Build history of the part. All positions in model axes, mm. A direction names the side the tool comes from. Round coordinates to 2 decimals unless told otherwise and drop trailing zeros. Write each loop counter-clockwise with the first axis right and the second up, starting at its lowest first coordinate (ties: lowest second). Pieces come first, ordered by that corner, then holes. Notation, with made-up numbers: M 30.25,32 L 59.25,32 A19 ccw 59.25,49 Z; hole C 5,88 d7. An arc over 180 degrees is marked long. Use a Markdown table: item, result.
Autodesk Inventor part; units mm, degrees
ref_plane "YZ Plane" through (0, 0, 0) normal (1, 0, 0) x (0, 1, 0)
ref_plane "XZ Plane" through (0, 0, 0) normal (0, 1, 0) x (-1, 0, 0)
ref_plane "XY Plane" through (0, 0, 0) normal (0, 0, 1) x (1, 0, 0)
sketch "スケッチ1" plane through (0, 0, 0) normal (0, 0, 1) x (1, 0, 0)
  line L0 (-24.2059, 21.7891) -> (-24.2059, -29.3158)
  line L1 (-24.2059, -29.3158) -> (21.4201, -29.3158)
  line L2 (21.4196, -22.9707) -> (21.4201, -22.9707)
  line L3 (-11.4832, -22.9707) -> (8.6224, -22.9707)
  arc A0 (-11.4832, -22.9707) -> (-19.2289, -15.2115) centre (-24.2804, -28) ccw
  line L4 (-19.2289, -15.2115) -> (-19.2289, -7.8183)
  arc A1 (-17.2289, -5.8183) -> (-19.2289, -7.8183) centre (-17.2289, -7.8183) ccw
  line L5 (-17.2289, -5.8183) -> (-11.461, -5.8183)
  arc A2 (-11.461, -5.8183) -> (-9.461, -3.8183) centre (-11.461, -3.8183) ccw
  line L6 (-9.461, -3.8183) -> (-9.461, 11.1956)
  arc A3 (-8.461, 12.1956) -> (-9.461, 11.1956) centre (-8.461, 11.1956) ccw
  line L7 (-8.461, 12.1956) -> (5.6023, 12.1956)
  arc A4 (6.6023, 11.1956) -> (5.6023, 12.1956) centre (5.6023, 11.1956) ccw
  line L8 (6.6023, 11.1956) -> (6.6023, -3.8183)
  arc A5 (6.6023, -3.8183) -> (8.6023, -5.8183) centre (8.6023, -3.8183) ccw
  line L9 (8.6023, -5.8183) -> (14.3681, -5.8183)
  arc A6 (16.3681, -7.8183) -> (14.3681, -5.8183) centre (14.3681, -7.8183) ccw
  line L10 (16.3681, -7.8183) -> (16.3681, -15.2115)
  arc A7 (16.3681, -15.2115) -> (8.6224, -22.9707) centre (21.4196, -28) ccw
  circle A8 centre (13.0661, -20.6138) radius 0.954
  circle A9 centre (-15.8899, -20.6138) radius 0.954
  arc A10 (-13.9359, 14.1081) -> (-14.9359, 13.1081) centre (-13.9359, 13.1081) ccw
  line L11 (-14.9359, 13.1081) -> (-14.9359, -0.6888)
  line L12 (-14.9359, -0.6888) -> (-19.2289, -0.6888)
  arc A11 (-5.7797, 14.1081) -> (-4.7797, 15.1081) centre (-5.7797, 15.1081) ccw
  line L13 (-5.7797, 14.1081) -> (-13.9359, 14.1081)
  line L14 (-24.2059, 26.7891) -> (-24.2059, 21.7891)
  line L15 (21.4201, -29.3158) -> (-24.2059, -29.3158)
  line L16 (-24.2059, -29.3158) -> (-24.2059, 26.7891)
  line L17 (21.4196, 26.7891) -> (21.4201, 26.7891)
  line L18 (-24.2059, 36.7891) -> (-24.2059, 26.7891)
  line L19 (-19.2289, 36.7891) -> (-24.2059, 36.7891)
  line L20 (-19.2289, 36.7891) -> (-19.2289, -0.6888)
  line L21 (-4.7797, 15.1081) -> (-4.7797, 36.7891)
  line L22 (21.4201, -29.3158) -> (21.4201, 36.7891)
  line L23 (21.4201, 36.7891) -> (-4.7797, 36.7891)
  line L24 (11.6885, 21.2661) -> (16.9518, 21.2661)
  line L25 (16.9518, 21.2661) -> (16.9518, -1.2633)
  line L26 (16.9518, -1.2633) -> (11.6885, -1.2633)
  line L27 (11.6885, -1.2633) -> (11.6885, 21.2661)
  point P0 (0, 0)
  point P1 (0, 0)
extrude "押し出し1" add sketch "スケッチ1" along normal blind 5
sketch "スケッチ2" plane through (0, 0, 0) normal (0, 0, -1) x (-1, 0, 0)
  line L0 (24.2059, 36.7891) -> (24.2059, -29.3158)
  line L1 (-21.4201, 36.7891) -> (24.2059, 36.7891)
  line L2 (24.2059, 36.7891) -> (24.2059, 31.7891)
  line L3 (24.2059, 31.7891) -> (-21.4201, 31.7891)
  line L4 (-21.4201, 31.7891) -> (-21.4201, 36.7891)
  point P0 (0, 0)
  dimension "d4" = 5
extrude "押し出し2" add sketch "スケッチ2" along normal blind 20
sketch "スケッチ3" plane through (-4.7797, 36.7891, 5) normal (0, 1, 0) x (1, 0, 0)
  line L0 (-10.1561, 5) -> (-14.4492, 5)
  line L1 (-14.4492, 5) -> (0, 5)
  line L2 (0, 5) -> (0, 12)
  line L3 (0, 12) -> (-14.4492, 12)
  line L4 (-14.4492, 12) -> (-14.4492, 5)
  point P0 (4.7797, 5)
  dimension "d7" = 7
extrude "押し出し3" cut sketch "スケッチ3" against normal blind 20
sketch "スケッチ4" plane through (-4.7797, 36.7891, 5) normal (0, 1, 0) x (1, 0, 0)
  circle A0 centre (-14.9262, 21) radius 1.75
  line L0 (-19.4262, 25) -> (26.1998, 25)
  line L1 (-19.4262, 25) -> (-19.4262, 0)
  circle A1 centre (21.6998, 21) radius 1.75
  line L2 (26.1998, 25) -> (26.1998, 0)
  circle A2 centre (21.6998, 15) radius 1.75
  circle A3 centre (-14.9262, 15) radius 1.75
  point P0 (4.7797, 5)
  dimension "d10" = 3.5
  dimension "d11" = 4
  dimension "d12" = 4.5
  dimension "d13" = 3.5
  dimension "d14" = 4
  dimension "d15" = 4.5
  dimension "d16" = 3.5
  dimension "d17" = 6
  dimension "d18" = 3.5
fillet "フィレット1" radius 2 2 edges at (-24.2059, -29.3158, 2.5) (21.4201, -29.3158, 2.5)
extrude "押し出し4" cut sketch "スケッチ4" against normal blind 20
chamfer "面取り1" distance 2 angle 45 2 edges at (8.3202, 31.7891, 0) (-21.7174, 31.7891, 0)
sketch "スケッチ5" plane through (-4.7797, 36.7891, 5) normal (0, 1, 0) x (1, 0, 0)
  circle A0 centre (21.6998, 15) radius 1.75
  circle A1 centre (-14.9262, 21) radius 1.75
  circle A2 centre (21.6998, 21) radius 1.75
  circle A3 centre (-14.9262, 15) radius 1.75
  line L0 (-14.4492, 12) -> (-14.4492, 0)
  line L1 (-14.4492, 12) -> (0, 12)
  line L2 (0, 12) -> (0, 0)
  line L3 (26.1998, 0) -> (0, 0)
  line L4 (26.1998, 25) -> (26.1998, 0)
  line L5 (-19.4262, 25) -> (26.1998, 25)
  line L6 (-19.4262, 25) -> (-19.4262, 0)
  line L7 (-14.4492, 0) -> (-19.4262, 0)
  point P0 (4.7797, 5)
properties part number "OpenMV-Mount-v2"
Q1. Cut at A-A on z = -10. Give the cut face in (x, y), and give its area (3 significant figures).
Response values:
| item | result |
|---|---|
| outline | M -24.21,31.79 L -21.46,31.79 L -21.46,36.79 L -24.21,36.79 Z; M -17.96,31.79 L 15.17,31.79 L 15.17,36.79 L -17.96,36.79 Z; M 18.67,31.79 L 21.42,31.79 L 21.42,36.79 L 18.67,36.79 Z |
| area | 193 mm2 |
Q2. Which spindle directions (+Z, -Z, +X, -X, +Y, -Y) get a long thin tool onto all of the face, cutting with end or side? Do faces 5 (the cylindrical face through (18.59, 34.32, -10.53)), 6 (the flat face through (-19.229, 18, 2)), 7 (the flat face through (16.368, -11, 2)), 8 (the flat face through (8, 1, 0)). Say none if no direction does.
Response values:
| item | result |
|---|---|
| face 5 | +Y, -Y |
| face 6 | +Z, +Y |
| face 7 | +Z, -Z |
| face 8 | -Z, +X, -X, -Y |
Q3. Two-plate mould, pull along Y, no slides. Class faces 1 (the flat face through (16.952, 10, 2)), 2 (the flat face through (-24.206, 14, 1)), 3 (the flat face through (14, 21.266, 2)), 4 (the flat face through (-21.68, 30.8, -1.01)): +Y half, -Y half, draft (parallel to the pull), parting line (faces both ways), or undercut.
Response values:
| item | result |
|---|---|
| face 1 | undercut |
| face 2 | draft |
| face 3 | undercut |
| face 4 | -Y half |
Q4. Cut at B-B on y = -13. Give the cut face in (x, z).
Response values:
| item | result |
|---|---|
| outline | M -24.21,0 L -19.23,0 L -19.23,5 L -24.21,5 Z; M 16.37,0 L 21.42,0 L 21.42,5 L 16.37,5 Z |
Q5. Cut at D-D on x = -4. Give the cut face in (y, z), and give its area (3 significant figures).
Response values:
| item | result |
|---|---|
| outline | M -29.32,0 L -22.97,0 L -22.97,5 L -29.32,5 Z; M 12.2,0 L 29.79,0 L 31.79,-2 L 31.79,-20 L 36.79,-20 L 36.79,5 L 12.2,5 Z |
| area | 257 mm2 |
Q6. Drill centre lines: L1, parallel to X at y = 34.7, z = -16; L2, parallel to X at y = 33.5, z = -15; L3, parallel to Y at x = 16, z = 3.5. Where is each one in solid material? Low to high.
Response values:
| item | result |
|---|---|
| L1 | x = -24.21 to -21.46, -17.96 to 15.17, 18.67 to 21.42 |
| L2 | x = -24.21 to -21.14, -18.27 to 15.48, 18.36 to 21.42 |
| L3 | y = -29.32 to -15.36, -6.66 to -1.26, 21.27 to 36.79 |
Q7. Cut at C-C on z = -4.25. Give the cut face in (x, y), and give its area (3 significant figures).
Response values:
| item | result |
|---|---|
| outline | M -24.21,31.79 L -19.23,31.79 L -19.23,36.79 L -24.21,36.79 Z; M -4.78,31.79 L 21.42,31.79 L 21.42,36.79 L -4.78,36.79 Z |
| area | 156 mm2 |
Q8. Drop flat-ended pins along their axis: P1, Ø23, axis at x = 5.5, y = -2, coming from the -Z side; P2, Ø9, axis at x = 5.5, z = -8, coming from the -Y side; P3, Ø1.3, axis at x = -16.5, z = 2.5, coming from the +Y side. Give the stop position or say it passes through.
Response values:
| item | result |
|---|---|
| P1 | stops at z = 0 |
| P2 | stops at y = 31.79 |
| P3 | stops at y = -0.69 |
